Can you work these out from the model? Positions are in its coordinate system, mm. A direction names the side the tool comes from. Give positions to 0.01 mm unless a question says otherwise; leave off trailing zeros. Put each result on its own line as item: value. Start each with the question number.
1) For faces 1 (the flat face through (-20, -1540, 2)), 2 (the flat face through (0, -20, 15)), 3 (the flat face through (0, -20, -15)), which set-ups out of +Z, -Z, +X, -X, +Y, -Y let a thin tool reach every point of the face, with its end or its side?
2) Please list where these lines run through material, in increasing order: line 1 along Z through (x, y) = (0, -39.3) (3 decimals); line 2 along Y through (x, z) = (546.5, -192); line 3 along Y through (x, z) = (651, -362). Write a range as from..to.
3) For P1, Ø1.5, axis at y = -38, z = 1.5, coming from the +X side; P2, Ø0.9, axis at y = -38.5, z = 0.5, coming from the -X side; P3, Ø15, axis at x = 1, z = 6.5, coming from the +Y side; P4, Ø6, axis at x = 582.5, y = -1346.5, coming from the +Z side, each with a flat end and sliding along its axis, tell me the tip position at first contact or that it passes through.
from build123d import *

# Parameters (mm, degrees)
F0_W      = 40
F0_H      = 30
F1_DEPTH  = 40
F3_R      = 14.5
F4_DEPTH  = 3
F5_W      = 8.5
F5_H      = 7.09
F6_DEPTH  = 3
F6_FACE_W = 8.5
F6_FACE_H = 7.09
F8_W      = 1593.75
F8_H      = 1329.375


with BuildPart() as f1:
    # F0 (on Front) → F1 (new body)
    with BuildSketch(Plane.XZ):
        Rectangle(F0_W, F0_H)
    extrude(amount=F1_DEPTH)

    # F3 (on face) → F4 (cut)
    with BuildSketch(Plane.XZ.offset(40)):
        Circle(F3_R)
    extrude(amount=-F4_DEPTH, mode=Mode.SUBTRACT)

    # F5 (on face) → F6 (join)
    with BuildSketch(Plane.XZ.offset(37)):
        Rectangle(F5_W, F5_H)
    extrude(amount=F6_DEPTH)

    # F6_face (on face) → F9 section 0
    with BuildSketch(Plane.XZ.offset(40)):
        Rectangle(F6_FACE_W, F6_FACE_H)
    # F8 (on offset) → F9 section 1
    with BuildSketch(Plane.XZ.offset(1540)):
        Rectangle(F8_W, F8_H)
    loft()

    # F10 (on face) → F11 (revolve)
    with BuildSketch(Plane.XZ):
        with BuildLine():
            ThreePointArc((0, -5), (5, 0), (0, 5))
            Line((0, 5), (0, -5))
        make_face()
    revolve(axis=Axis((0, 0, 0), (0, 0, -1)))


solid = f1.part
Recorded:
1. face 1: +Z, -Z, +X, -X, -Y
1. face 2: +Z, +X, -X, +Y
1. face 3: -Z, +X, -X, +Y
2. line 1: -15..-14.5, -3.545..3.545, 14.5..15
2. line 2: -1540..-1066.18
2. line 3: -1540..-1263.94
3. P1: x = 20
3. P2: x = -20
3. P3: y = 5
3. P4: z = 580.72
